from build123d import *

# Parameters (mm, degrees)
SKETCH2_R           = 3.2
BOSS_EXTRUDE1_DEPTH = 10
FILLET1_R           = 1
SKETCH3_R           = 3.2
CUT_EXTRUDE1_DEPTH  = 40


with BuildPart() as part:
    # Sketch2 → Boss-Extrude1 (new body)
    with BuildSketch(Plane(origin=(0, 0, 0), x_dir=(1, 0, 0), z_dir=(0, 1, 0))):
        with BuildLine():
            Line((-2, 44.955533586), (-20.57248383, 28.315594803))
            Line((-20.57248383, 28.315594803), (-26.450336353, 36.405764747))
            ThreePointArc((-26.450336353, 36.405764747), (-27.253018295, 35.808839605), (-28.04223364, 35.194220158))
            Line((-28.04223364, 35.194220158), (-33.28697807, 10.815594803))
            Line((-33.28697807, 10.815594803), (-42.797543233, 13.905764747))
            ThreePointArc((-42.797543233, 13.905764747), (-43.09606277, 12.951037555), (-43.373287149, 11.989910837))
            Line((-43.373287149, 11.989910837), (-33.28697807, -10.815594803))
            Line((-33.28697807, -10.815594803), (-42.797543233, -13.905764747))
            ThreePointArc((-42.797543233, -13.905764747), (-42.477876048, -14.853620651), (-42.137219172, -15.794136902))
            Line((-42.137219172, -15.794136902), (-20.57248383, -28.315594803))
            Line((-20.57248383, -28.315594803), (-26.450336353, -36.405764747))
            ThreePointArc((-26.450336353, -36.405764747), (-25.634584446, -36.984700625), (-24.806165662, -37.545361167))
            Line((-24.806165662, -37.545361167), (0, -35))
            Line((0, -35), (0, -45))
            ThreePointArc((0, -45), (1.000247127, -44.988882023), (2, -44.955533586))
            Line((2, -44.955533586), (20.57248383, -28.315594803))
            Line((20.57248383, -28.315594803), (26.450336353, -36.405764747))
            ThreePointArc((26.450336353, -36.405764747), (27.253018295, -35.808839605), (28.04223364, -35.194220158))
            Line((28.04223364, -35.194220158), (33.28697807, -10.815594803))
            Line((33.28697807, -10.815594803), (42.797543233, -13.905764747))
            ThreePointArc((42.797543233, -13.905764747), (43.09606277, -12.951037555), (43.373287149, -11.989910837))
            Line((43.373287149, -11.989910837), (33.28697807, 10.815594803))
            Line((33.28697807, 10.815594803), (42.797543233, 13.905764747))
            ThreePointArc((42.797543233, 13.905764747), (42.477876048, 14.853620651), (42.137219172, 15.794136902))
            Line((42.137219172, 15.794136902), (20.57248383, 28.315594803))
            Line((20.57248383, 28.315594803), (26.450336353, 36.405764747))
            ThreePointArc((26.450336353, 36.405764747), (25.634584446, 36.984700625), (24.806165662, 37.545361167))
            Line((24.806165662, 37.545361167), (0, 35))
            Line((0, 35), (0, 45))
            ThreePointArc((0, 45), (-1.000247127, 44.988882023), (-2, 44.955533586))
        make_face()
        with Locations(Location((0, 0, 0), (0, 0, 270))):
            Circle(SKETCH2_R, mode=Mode.SUBTRACT)
    extrude(amount=BOSS_EXTRUDE1_DEPTH)

    # Fillet1
    fillet1_edges = [part.edges().sort_by_distance(p)[0] for p in [
        (-20.57248383, 5, 28.315594803),
        (-33.28697807, 5, 10.815594803),
        (-33.28697807, 5, -10.815594803),
        (-20.57248383, 5, -28.315594803),
        (0, 5, -35),
        (20.57248383, 5, -28.315594803),
        (33.28697807, 5, -10.815594803),
        (33.28697807, 5, 10.815594803),
        (20.57248383, 5, 28.315594803),
        (0, 5, 35),
    ]]
    fillet(fillet1_edges, radius=FILLET1_R)

    # Sketch3 → Cut-Extrude1 (cut)
    with BuildSketch(Plane(origin=(352.77049505, 10, -1092.526706597), x_dir=(-0.9455896889977465, 0, 0.32536155283183854), z_dir=(0, 1, 0))):
        with Locations(Location((697.366992794, 931.392438652, 0), (0, 0, 71.012519009))):
            Circle(SKETCH3_R)
    extrude(amount=-CUT_EXTRUDE1_DEPTH, mode=Mode.SUBTRACT)


solid = part.part
Can you work these out from the model? Positions are in its coordinate system, mm. A direction names the side the tool comes from. Give positions to 0.01 mm unless a question says otherwise; leave off trailing zeros. Write each loop counter-clockwise with the first axis right and the second up, starting at its lowest first coordinate (ties: lowest second). Pieces come first, ordered by that corner, then holes. Notation, with made-up numbers: M 32.5,-7 L 57.5,-7 A26 ccw 57.5,11 Z; hole C 21.25,78 d6. An arc over 180 degrees is marked long. Answer in a Markdown table with one row per item. Add a question column.
Item 1: Imagine slicing it at B-B, the plane x = -5. Write out the boundary of the cut face in (y, z), plus the area to 3 significant figures.
Item 2: For pin 1 Ø2 at (x, y) = (23, 5.5) entering from -Z; pin 2 Ø1 at (x, z) = (-19.5, -32.5) entering from -Y; pin 3 Ø4.5 at (y, z) = (6.5, -40) entering from +X; pin 4 Ø6 at (x, y) = (-10, 4.5) entering from +Z, each with a flat end and sliding along its axis, tell me the tip position at first contact or that it passes through.
Item 3: Imagine slicing it at C-C, the plane y = 7. State how many separate pieces and enclosed holes the cut face has, plus the area to 3 significant figures.
Item 4: Imagine slicing it at D-D, the plane x = -15. Write out the boundary of the cut face in (y, z).
Item 5: Please list where these lines run through material, in increasing order: L1, parallel to X at y = 6, z = 29; L2, parallel to X at y = 1.5, z = 0; L3, parallel to Z at x = -25, y = 2.75.
Item 6: We'd pull the mould along Z, two halves only. Please class faces 1 (the flat face through (-31.98, 4.93, 21.69)), 2 (the flat face through (0, 5, 40)), 3 (the flat face through (-10.749, 4.93, -37.117)): released by +Z, released by -Z, zero draft, split by the parting line, or undercut.
Item 7: Imagine slicing it at A-A, the plane z = 0. Write out the boundary of the cut face in (x, y), plus the area to 3 significant figures.
Item 8: On a 3-axis mill with a long thin cutter (end or side, diameter ignored), from which of +Z, -Z, +X, -X, +Y, -Y can I reach the whole of each face in a straight line? I mean faces 4 (the flat face through (-13.12, 4.93, 36.346)), 5 (the flat face through (0, 5, -40)), 6 (the flat face through (-38.51, 4.93, 12.513)). Say none if no direction works.
Evaluation:
| question | item | result |
|---|---|---|
| 1 | outline | M 0,-42.27 L 10,-42.27 L 10,12.2 L 0,12.2 Z; M 0,17.97 L 10,17.97 L 10,35.51 L 0,35.51 Z |
| 1 | area | 720 mm² |
| 2 | pin 1 | stops at z = -37.46 |
| 2 | pin 2 | passes through |
| 2 | pin 3 | stops at x = 0 |
| 2 | pin 4 | stops at z = 36.33 |
| 3 | separate pieces | 1 |
| 3 | enclosed holes | 2 |
| 3 | area | 4,730 mm² |
| 4 | outline | M 0,-33.31 L 10,-33.31 L 10,36.54 L 0,36.54 Z |
| 5 | L1 | x = -21.11 to 19.81, 21.02 to 29.37 |
| 5 | L2 | x = -38.07 to -3.2, 3.2 to 38.07 |
| 5 | L3 | z = -34.41 to 25.74, 34.41 to 37.42 |
| 6 | face 1 | undercut |
| 6 | face 2 | zero draft |
| 6 | face 3 | released by -Z |
| 7 | outline | M -38.07,0 L -3.2,0 L -3.2,10 L -38.07,10 Z; M 3.2,0 L 38.07,0 L 38.07,10 L 3.2,10 Z |
| 7 | area | 697 mm² |
| 8 | face 4 | +Z, +Y, -Y |
| 8 | face 5 | -Z, +Y, -Y |
| 8 | face 6 | -X, +Y, -Y |
